Design review of the part built by this model. Coordinates are the model's own, in mm. Face numbers are marked on the shaded views. A direction names the side the tool comes from. Coordinates: 2 decimals unless noted, no trailing zeros. Loops run counter-clockwise (first coordinate to the right, second up) from the corner with the lowest first, then second, coordinate; pieces in that order, holes last. Notation, with made-up numbers: M 42.5,89 L 61.5,89 A24 ccw 61.5,122 Z; hole C 77,48.5 d4. An arc over 180 degrees is marked long. One line per item, written item: value.
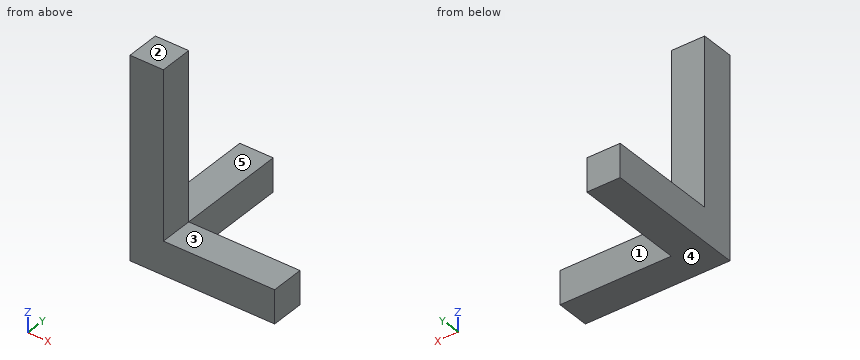
```python
from build123d import *

# Parameters (mm, degrees)
SKETCH1_W           = 3
SKETCH1_H           = 3
BOSS_EXTRUDE2_DEPTH = 15
SKETCH2_W           = 3
SKETCH2_H           = 3
BOSS_EXTRUDE3_DEPTH = 10
SKETCH3_W           = 3
SKETCH3_H           = 3
BOSS_EXTRUDE4_DEPTH = 10
SKETCH4_W           = 3
SKETCH4_H           = 3
BOSS_EXTRUDE5_DEPTH = 15
SKETCH1_2_W         = 3
SKETCH1_2_H         = 3
CUT_EXTRUDE1_DEPTH  = 12


with BuildPart() as part:
    # Sketch1 → Boss-Extrude2 (new body)
    with BuildSketch(Plane.XY):
        Rectangle(SKETCH1_W, SKETCH1_H)
    extrude(amount=BOSS_EXTRUDE2_DEPTH)

    # Sketch2 → Boss-Extrude3 (add)
    with BuildSketch(Plane(origin=(1.5, 0, 0), x_dir=(0, 0, -1), z_dir=(1, 0, 0))):
        with Locations((-13.5, 0)):
            Rectangle(SKETCH2_W, SKETCH2_H)
    extrude(amount=BOSS_EXTRUDE3_DEPTH)

    # Sketch3 → Boss-Extrude4 (add)
    with BuildSketch(Plane(origin=(0, 1.5, 0), x_dir=(1, 0, 0), z_dir=(0, 1, 0))):
        with Locations((0, -13.5)):
            Rectangle(SKETCH3_W, SKETCH3_H)
    extrude(amount=BOSS_EXTRUDE4_DEPTH)

    # Sketch4 → Boss-Extrude5 (add)
    with BuildSketch(Plane.XY.offset(15)):
        Rectangle(SKETCH4_W, SKETCH4_H)
    extrude(amount=BOSS_EXTRUDE5_DEPTH)

    # Sketch1<2> → Cut-Extrude1 (cut)
    with BuildSketch(Plane.XY):
        Rectangle(SKETCH1_2_W, SKETCH1_2_H)
    extrude(amount=CUT_EXTRUDE1_DEPTH, mode=Mode.SUBTRACT)


solid = part.part
```
(1) Tool access review of the marked faces 1, 2, 3, 4 and 5: name each direction out of +Z, -Z, +X, -X, +Y, -Y from which nothing blocks a thin tool from reaching the whole face with its end or side.
Reply:
face 1: +Z, -Z, +X, +Y
face 2: +Z, +X, -X, +Y, -Y
face 3: +Z, +X, +Y, -Y
face 4: -Z, +X, -X, +Y, -Y
face 5: +Z, +X, -X, +Y
(2) We need section A-A on z = 14.5. State the section outline as (x, y) points, then the cut area to 3 significant figures.
Reply:
outline: M -1.5,-1.5 L 11.5,-1.5 L 11.5,1.5 L 1.5,1.5 L 1.5,11.5 L -1.5,11.5 Z
area: 69.0 mm2
(3) We need section D-D on z = 17.25. State the section outline as (x, y) points, then the cut area to 3 significant figures.
Reply:
outline: M -1.5,-1.5 L 1.5,-1.5 L 1.5,1.5 L -1.5,1.5 Z
area: 9.00 mm2
(4) Insertion check: pin 1 (2.5 mm diameter, centred on x = 4.5, y = 0, fed in from +Z); pin 2 (0.9 mm diameter, centred on y = -0.5, z = 25.5, fed in from +X); pin 3 (2.5 mm diameter, centred on x = 0, z = 21.5, fed in from +Y). Each pin has a flat end and moves straight along its axis. Give the tip position at first contact, or say it passes through.
Reply:
pin 1: stops at z = 15
pin 2: stops at x = 1.5
pin 3: stops at y = 1.5
(5) To check wall thickness, follow line 1 along Y through (x, z) = (10, 13.75); line 2 along Z through (x, y) = (-0.5, 7.5). State the ranges of each line that lie inside material, in increasing order. Write a range as [from, to].
Reply:
line 1: y = [-1.5, 1.5]
line 2: z = [12, 15]
(6) We need section B-B on y = 0.25. State the section outline as (x, z) points.
Reply:
outline: M -1.5,12 L 11.5,12 L 11.5,15 L 1.5,15 L 1.5,30 L -1.5,30 Z
(7) We need section C-C on x = 2.25. State the section outline as (y, z) points, then the cut area to 3 significant figures.
Reply:
outline: M -1.5,12 L 1.5,12 L 1.5,15 L -1.5,15 Z
area: 9.00 mm2
